Geometry check sheet. Reference: the model listing, model coordinates, mm. Face numbers are marked on the shaded views. A direction names the side the tool comes from. Give positions to 0.01 mm unless a question says otherwise; leave off trailing zeros. Write each loop counter-clockwise with the first axis right and the second up, starting at its lowest first coordinate (ties: lowest second). Pieces come first, ordered by that corner, then holes. Notation, with made-up numbers: M 73.25,17 L 80.25,17 A13 cw 80.25,34 Z; hole C 24,3.5 d11. An arc over 180 degrees is marked long. Write each question's results on one line, items separated by ' | '.
```python
from build123d import *

# Parameters (mm, degrees)
SKETCH_1_R           = 16.5
SKETCH_1_R_2         = 14
EXTRUDE_1_DEPTH      = 30
EXTRUDE_2_DEPTH      = 30
EXTRUDE_2_DEPTH_BACK = 30
SKETCH_3_R           = 14
CUT_EXTRUDE_1_DEPTH  = 50
SKETCH_4_R           = 2.5
CUT_EXTRUDE_2_DEPTH  = 56


with BuildPart() as part:
    # Sketch 1 → Extrude 1 (new body)
    with BuildSketch(Plane(origin=(0, 0, 0), x_dir=(1, 0, 0), z_dir=(0, 1, 0))):
        Circle(SKETCH_1_R)
        Circle(SKETCH_1_R_2, mode=Mode.SUBTRACT)
    extrude(amount=EXTRUDE_1_DEPTH)

    # Sketch 2 → Extrude 2 (add, two sides)
    with BuildSketch(Plane.XY) as extrude_2_sk:
        Polygon((27.5, 30), (-27.5, 30), (-27.5, 68), (-25.5, 68), (-25.5, 32), (25.5, 32), (25.5, 68), (27.5, 68), align=None)
    extrude(amount=EXTRUDE_2_DEPTH)
    extrude(extrude_2_sk.sketch, amount=-EXTRUDE_2_DEPTH_BACK)

    # Sketch 3 → Cut-Extrude 1 (cut)
    with BuildSketch(Plane.XZ.offset(-30)):
        Circle(SKETCH_3_R)
    extrude(amount=-CUT_EXTRUDE_1_DEPTH, mode=Mode.SUBTRACT)

    # Sketch 4 → Cut-Extrude 2 (cut, through all)
    with BuildSketch(Plane(origin=(27.5, 0, 0), x_dir=(0, 0, -1), z_dir=(1, 0, 0))):
        with Locations((0, 50)):
            Circle(SKETCH_4_R)
        with Locations((0, 15)):
            Circle(SKETCH_4_R)
        Polygon((-30, 38), (-30, 68), (-10, 68), align=None)
        Polygon((30, 68), (10, 68), (30, 38), align=None)
    extrude(amount=-CUT_EXTRUDE_2_DEPTH, mode=Mode.SUBTRACT)


solid = part.part
```
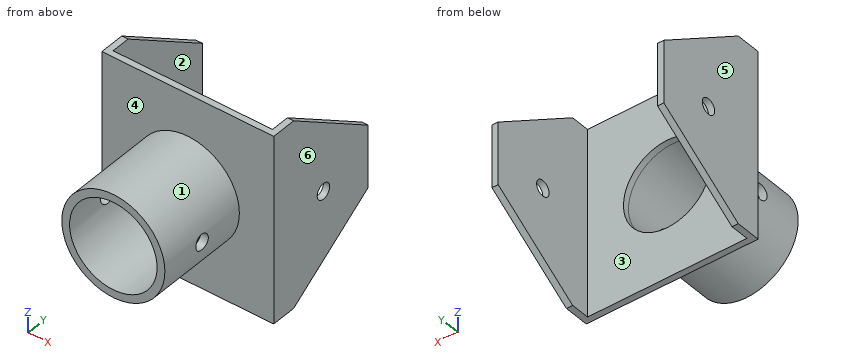
Q1. Depth check by flat-ended pin: P1, Ø10, axis at y = 13.5, z = -17.5, coming from the +X side; P2, Ø8, axis at x = 17.5, y = 19, coming from the +Z side. Enter the tip coordinate at first touch or a pass-through.
Answer key:
P1: stops at x = 10.77 | P2: stops at z = 9.49
Q2. Access from +Z, -Z, +X, -X, +Y, -Y to the whole of each face (thin tool, end or side, straight path). Record for the marked faces 1 and 2.
Answer key:
face 1: -Y | face 2: +Z, -Z, +Y
Q3. Section check C-C (y = 50). Enter the section's corners in (x, z).
Answer key:
outline: M -27.5,-22 L -25.5,-22 L -25.5,-2.5 L -27.5,-2.5 Z; M -27.5,2.5 L -25.5,2.5 L -25.5,22 L -27.5,22 Z; M 25.5,-22 L 27.5,-22 L 27.5,-2.5 L 25.5,-2.5 Z; M 25.5,2.5 L 27.5,2.5 L 27.5,22 L 25.5,22 Z
Q4. Material ranges on probe 1 along Y at (x, z) = (-26, 0); probe 2 along X at (y, z) = (33.5, 25); probe 3 along Y at (x, z) = (15.55, 0), recorded low to high. Write a range as [from, to].
Answer key:
probe 1: y = [30, 47.5], [52.5, 68] | probe 2: x = [-27.5, -25.5], [25.5, 27.5] | probe 3: y = [0, 12.5], [17.5, 32]
Q5. Section check B-B (z = 0). State how many separate pieces and enclosed holes the cut face has, then the cut area to 3 significant figures.
Answer key:
separate pieces: 6 | enclosed holes: 0 | area: 303 mm2
Q6. Section check A-A (x = 0). Enter the section's corners in (y, z), then the cut area to 3 significant figures.
Answer key:
outline: M 0,-16.5 L 30,-16.5 L 30,-30 L 32,-30 L 32,-14 L 0,-14 Z; M 0,14 L 32,14 L 32,30 L 30,30 L 30,16.5 L 0,16.5 Z | area: 214 mm2
Q7. Release check for a two-part mould opening along X. For the marked faces 3, 4, 5 and 6 record: released by +X, released by -X, zero draft, split by the parting line, or undercut.
Answer key:
face 3: undercut | face 4: zero draft | face 5: released by -X | face 6: released by +X
Q8. Section check D-D (y = 15). Enter the section's corners in (x, z), then the cut area to 3 significant figures.
Answer key:
outline: M -16.31,-2.5 A16.5 ccw 16.31,-2.5 L 13.77,-2.5 A14 cw -13.77,-2.5 Z; M -16.31,2.5 L -13.77,2.5 A14 cw 13.77,2.5 L 16.31,2.5 A16.5 ccw Z | area: 214 mm2
